from build123d import *

# Parameters (mm, degrees)
BASENUT_DEPTH = 16
DOMEFILLET_R  = 1


with BuildPart() as part:
    # BaseNutSke → BaseNut (new body)
    with BuildSketch(Plane(origin=(0, 0, 0), x_dir=(0, 0, -1), z_dir=(1, 0, 0))):
        Polygon((15, 8.660254038), (15, -8.660254038), (0, -17.320508076), (-15, -8.660254038), (-15, 8.660254038), (0, 17.320508076), align=None)
    extrude(amount=BASENUT_DEPTH)

    # DomeSke → Dome (revolve)
    with BuildSketch(Plane.XY, mode=Mode.PRIVATE) as dome_sk:
        with BuildLine():
            Line((34, 0), (0, 0))
            Line((0, 0), (0, 14))
            Line((0, 14), (20, 14))
            ThreePointArc((20, 14), (29.899494937, 9.899494937), (34, 0))
        make_face()
    revolve(dome_sk.sketch.rotate(Axis((0, 0, 0), (1, 0, 0)), 90), axis=Axis((0, 0, 0), (1, 0, 0)))

    # Sketch4 → DoubleChamfer (revolve, cut)
    with BuildSketch(Plane.XY):
        Polygon((0, 15), (2.783121635, 19.820508076), (13.216878365, 19.820508076), (16, 15), (18, 15), (18, 30), (-2, 30), (-2, 15), align=None)
    revolve(axis=Axis((0, 0, 0), (1, 0, 0)), mode=Mode.SUBTRACT)

    # TapDriSke → TapDrill (revolve, cut)
    with BuildSketch(Plane.XY, mode=Mode.PRIVATE) as tapdrill_sk:
        Polygon((0, 8.75), (23, 8.75), (28.257530416, 0), (0, 0), align=None)
    revolve(tapdrill_sk.sketch.rotate(Axis((0, 0, 0), (1, 0, 0)), 90), axis=Axis((0, 0, 0), (1, 0, 0)), mode=Mode.SUBTRACT)

    # UcutSke → Undercut (revolve, cut)
    with BuildSketch(Plane.XY, mode=Mode.PRIVATE) as undercut_sk:
        Polygon((17.899422863, 10.1), (17.12, 8.75), (17.12, 0.25), (26.42, 0.25), (26.42, 10.1), align=None)
    revolve(undercut_sk.sketch.rotate(Axis((0, 0, 0), (1, 0, 0)), 90), axis=Axis((0, 0, 0), (1, 0, 0)), mode=Mode.SUBTRACT)

    # EndChamferSketch → EndChamfer (revolve, cut)
    with BuildSketch(Plane.XY):
        Polygon((-0.0254, 10), (0.0254, 10), (0.988185365, 8.625), (-0.0254, 8.625), align=None)
    revolve(axis=Axis((0, 0, 0), (-1, 0, 0)), mode=Mode.SUBTRACT)

    # DomeFillet
    domefillet_edges = [part.edges().sort_by_distance(p)[0] for p in [
        (16, 0, -14),
    ]]
    fillet(domefillet_edges, radius=DOMEFILLET_R - 0.0001)  # a hair under: the kernel refuses the full size


solid = part.part
For this review, take the finished solid that the model builds, in its own axes (mm). Round coordinates to 2 decimals unless told otherwise and drop trailing zeros. Write each loop counter-clockwise with the first axis right and the second up, starting at its lowest first coordinate (ties: lowest second). Pieces come first, ordered by that corner, then holes. Notation, with made-up numbers: M -27,38.25 L 7,38.25 A32 ccw 7,66.25 Z; hole C 72,54 d9. An arc over 180 degrees is marked long. Write item = value, one per line. Start each with the question number.
(1) For line 1 along Z through (x, y) = (17.5, -0.5); line 2 along Y through (x, z) = (11, 5); line 3 along Y through (x, z) = (24.5, 1), list the stretches that pass through material, from the lowest coordinate up.
(2) We need section C-C (x = 24.5). Give the boundary of the cut face in (y, z), then the cut area to 3 significant figures.
(3) The part is to be moulded in two halves that separate along X. For faces 1 (the face through (26.42, -2.4, 2.4)), 2 (the face through (9.12, 8.54, -1.9)), 3 (the face through (15.68, 7.74, -13.49)), say which applies: +X half, -X half, draft (parallel to the pull), parting line (faces both ways), or undercut.
(4) We need section A-A (x = 12). Give the boundary of the cut face in (y, z).
(5) We need section B-B (x = 31). Give the boundary of the cut face in (y, z), then the cut area to 3 significant figures.
(6) Clearance check with flat-ended pins moving along their axes: pin 1 Ø18 at (y, z) = (0, 0) entering from -X; pin 2 Ø6 at (x, y) = (22.5, -4.5) entering from +Z; pin 3 Ø1 at (x, y) = (30.5, 2) entering from +Z. State where each tip first meets the part, or that it passes through.
Results found:
q1.line_1 = -13.99 to -9.39, 9.39 to 13.99
q1.line_2 = -14.43 to -7.18, 7.18 to 14.43
q1.line_3 = -13.22 to -10.05, 10.05 to 13.22
q2.outline = C 0,0 d26.51; hole C 0,0 d20.2
q2.area = 232 mm²
q3.face_1 = undercut
q3.face_2 = draft
q3.face_3 = +X half
q4.outline = M -17.32,0 L -8.66,-15 L 8.66,-15 L 17.32,0 L 8.66,15 L -8.66,15 Z; hole C 0,0 d17.5
q5.outline = C 0,0 d17.32
q5.area = 236 mm²
q6.pin_1 = 0.73
q6.pin_2 = 13.83
q6.pin_3 = 9.6
